from build123d import *

# Parameters (mm, degrees)
F1_DEPTH = 5
F3_DEPTH = 10
F5_DEPTH = 25


with BuildPart() as f1:
    # F0 (on Front) → F1 (new body)
    with BuildSketch(Plane.XZ):
        with BuildLine():
            Line((32.2, -24), (32.2, 24))
            Line((32.2, 24), (6.5, 24))
            Line((6.5, 24), (6.5, 10.8))
            Line((6.5, 10.8), (8.4, 10.8))
            Line((8.4, 10.8), (8.4, 14.8))
            ThreePointArc((8.4, 14.8), (14.9, 21.3), (21.4, 14.8))
            Line((21.4, 14.8), (21.4, 10.8))
            Line((21.4, 10.8), (24.4, 10.8))
            Line((24.4, 10.8), (24.4, -10.8))
            Line((24.4, -10.8), (21.4, -10.8))
            Line((21.4, -10.8), (21.4, -14.8))
            ThreePointArc((21.4, -14.8), (14.9, -21.3), (8.4, -14.8))
            Line((8.4, -14.8), (8.4, -10.8))
            Line((8.4, -10.8), (-8.4, -10.8))
            Line((-8.4, -10.8), (-8.4, -14.8))
            ThreePointArc((-8.4, -14.8), (-14.9, -21.3), (-21.4, -14.8))
            Line((-21.4, -14.8), (-21.4, -10.8))
            Line((-21.4, -10.8), (-24.4, -10.8))
            Line((-24.4, -10.8), (-24.4, 10.8))
            Line((-24.4, 10.8), (-21.4, 10.8))
            Line((-21.4, 10.8), (-21.4, 14.8))
            ThreePointArc((-21.4, 14.8), (-14.9, 21.3), (-8.4, 14.8))
            Line((-8.4, 14.8), (-8.4, 10.8))
            Line((-8.4, 10.8), (-6.5, 10.8))
            Line((-6.5, 10.8), (-6.5, 24))
            Line((-6.5, 24), (-32.2, 24))
            Line((-32.2, 24), (-32.2, -24))
            Line((-32.2, -24), (32.2, -24))
        make_face()
    extrude(amount=F1_DEPTH)

    # F2 (on face) → F3 (join)
    with BuildSketch(Plane(origin=(0, 0, 0), x_dir=(-1, 0, 0), z_dir=(0, 1, 0))):
        with BuildLine():
            Line((24.4, 10.8), (24.4, -10.8))
            Line((24.4, -10.8), (21.4, -10.8))
            Line((21.4, -10.8), (21.4, -14.8))
            ThreePointArc((21.4, -14.8), (14.9, -21.3), (8.4, -14.8))
            Line((8.4, -14.8), (8.4, -10.8))
            Line((8.4, -10.8), (-8.4, -10.8))
            Line((-8.4, -10.8), (-8.4, -14.8))
            ThreePointArc((-8.4, -14.8), (-14.9, -21.3), (-21.4, -14.8))
            Line((-21.4, -14.8), (-21.4, -10.8))
            Line((-21.4, -10.8), (-24.4, -10.8))
            Line((-24.4, -10.8), (-24.4, 10.8))
            Line((-24.4, 10.8), (-21.4, 10.8))
            Line((-21.4, 10.8), (-21.4, 14.8))
            ThreePointArc((-21.4, 14.8), (-14.9, 21.3), (-8.4, 14.8))
            Line((-8.4, 14.8), (-8.4, 10.8))
            Line((-8.4, 10.8), (-6.5, 10.8))
            Line((-6.5, 10.8), (-6.5, 24))
            Line((-6.5, 24), (-32.2, 24))
            Line((-32.2, 24), (-32.2, -24))
            Line((-32.2, -24), (32.2, -24))
            Line((32.2, -24), (32.2, 24))
            Line((32.2, 24), (6.5, 24))
            Line((6.5, 24), (6.5, 10.8))
            Line((6.5, 10.8), (8.4, 10.8))
            Line((8.4, 10.8), (8.4, 14.8))
            ThreePointArc((8.4, 14.8), (14.9, 21.3), (21.4, 14.8))
            Line((21.4, 14.8), (21.4, 10.8))
            Line((21.4, 10.8), (24.4, 10.8))
        make_face()
        with BuildLine():
            Line((21.4, -14.8), (21.4, -10.8))
            Line((21.4, -10.8), (8.4, -10.8))
            Line((8.4, -10.8), (8.4, -14.8))
            ThreePointArc((8.4, -14.8), (14.9, -21.3), (21.4, -14.8))
        make_face()
        with BuildLine():
            Line((-8.4, -14.8), (-8.4, -10.8))
            Line((-8.4, -10.8), (-21.4, -10.8))
            Line((-21.4, -10.8), (-21.4, -14.8))
            ThreePointArc((-21.4, -14.8), (-14.9, -21.3), (-8.4, -14.8))
        make_face()
        with BuildLine():
            Line((8.4, 10.8), (21.4, 10.8))
            Line((21.4, 10.8), (21.4, 14.8))
            ThreePointArc((21.4, 14.8), (14.9, 21.3), (8.4, 14.8))
            Line((8.4, 14.8), (8.4, 10.8))
        make_face()
        with BuildLine():
            Line((-21.4, 10.8), (-8.4, 10.8))
            Line((-8.4, 10.8), (-8.4, 14.8))
            ThreePointArc((-8.4, 14.8), (-14.9, 21.3), (-21.4, 14.8))
            Line((-21.4, 14.8), (-21.4, 10.8))
        make_face()
    extrude(amount=F3_DEPTH)

    # F4 (on face) → F5 (join)
    with BuildSketch(Plane(origin=(0, 10, 0), x_dir=(-1, 0, 0), z_dir=(0, 1, 0))):
        Polygon((32.2, -24), (32.2, 24), (6.5, 24), (6.5, 10.8), (24.4, 10.8), (24.4, -10.8), (-24.4, -10.8), (-24.4, 10.8), (-6.5, 10.8), (-6.5, 24), (-32.2, 24), (-32.2, -24), align=None)
        Polygon((6.5, 10.8), (6.5, 24), (-6.5, 24), (-6.5, 10.8), (-24.4, 10.8), (-24.4, -10.8), (24.4, -10.8), (24.4, 10.8), align=None)
        with BuildLine():
            ThreePointArc((5.5288725662, 5.5), (16.8680666762, 9.6842239514), (24.1, 0))
            ThreePointArc((24.1, 0), (16.8680666762, -9.6842239514), (5.5288725662, -5.5))
            Line((5.5288725662, -5.5), (0, -5.5))
            Line((0, -5.5), (-5.5288725662, -5.5))
            ThreePointArc((-5.5288725662, -5.5), (-24.1, 0), (-5.5288725662, 5.5))
            Line((-5.5288725662, 5.5), (0, 5.5))
            Line((0, 5.5), (5.5288725662, 5.5))
        make_face(mode=Mode.SUBTRACT)
    extrude(amount=F5_DEPTH)


solid = f1.part
Work out the finished part from the listing and answer in its coordinate system (mm). A direction names the side the tool comes from. Give positions to 0.01 mm unless a question says otherwise; leave off trailing zeros. Loops run counter-clockwise (first coordinate to the right, second up) from the corner with the lowest first, then second, coordinate; pieces in that order, holes last. Notation, with made-up numbers: (-34, 18.25) - (15, 18.25) arc R18 cw to (15, 50.25) - close; hole circle Ø2 at (35, 49.5). An arc over 180 degrees is marked (long way). Answer in a Markdown table with one row per item. Add a question column.
Q1. The part is cut by section C-C (x = 19.5). Determine the outline of the cut face in (y, z).
Q2. The part is cut by section D-D (y = 7). Determine the outline of the cut face in (x, z).
Q3. A tool of negligible diameter and unlimited length cuts with its end or side. For faces 3 (the flat face through (0, 22, -5.5)), 4 (the flat face through (-15, 0, 15)), 5 (the flat face through (-32.2, 15, 0)), from which of +Z, -Z, +X, -X, +Y, -Y can it reach the whole face along a straight path? Write none if from no direction.
Q4. Consider line 1 along X through (y, z) = (2, 9.5); line 2 along X through (y, z) = (23.5, 0); line 3 along Z through (x, y) = (14, 15). Determine where each line is inside the solid, lowest interval first.
Q5. This flat-tipped pin is pushed along its axis until it touches: P1, Ø5, axis at x = 12, z = -15, coming from the -Y side. Where does it stop, or does it pass through?
Q6. Determine the mould class of faces 1 (the flat face through (21.4, -2, -13)), 2 (the flat face through (-8, -5, 11)) for opening direction Z: released by +Z, released by -Z, zero draft, split by the parting line, or undercut.
Q7. The part is cut by section A-A (y = 26). Determine the outline of the cut face in (x, z).
Q8. The part is cut by section B-B (z = 8.5). Determine the outline of the cut face in (x, y).
Solution:
| question | item | result |
|---|---|---|
| 1 | outline | (-5, -24) - (35, -24) - (35, -8.47) - (10, -8.47) - (10, -10.8) - (0, -10.8) - (0, -19.39) - (-5, -19.39) - close; (-5, 19.39) - (0, 19.39) - (0, 10.8) - (10, 10.8) - (10, 8.47) - (35, 8.47) - (35, 24) - (-5, 24) - close |
| 2 | outline | (-32.2, -24) - (32.2, -24) - (32.2, 24) - (6.5, 24) - (6.5, 10.8) - (24.4, 10.8) - (24.4, -10.8) - (-24.4, -10.8) - (-24.4, 10.8) - (-6.5, 10.8) - (-6.5, 24) - (-32.2, 24) - close |
| 3 | face 3 | +Y, -Y |
| 3 | face 4 | -Y |
| 3 | face 5 | +Z, -Z, -X, +Y, -Y |
| 4 | line 1 | x = -32.2 to -24.4, 24.4 to 32.2 |
| 4 | line 2 | x = -32.2 to -24.1, 24.1 to 32.2 |
| 4 | line 3 | z = -24 to -10.1, 10.1 to 24 |
| 5 | P1 | stops at y = 0 |
| 6 | face 1 | undercut |
| 6 | face 2 | zero draft |
| 7 | outline | (-32.2, -24) - (32.2, -24) - (32.2, 24) - (-32.2, 24) - close; hole (-5.53, -5.5) - (5.53, -5.5) arc R10.1 ccw (long way) to (5.53, 5.5) - (-5.53, 5.5) arc R10.1 ccw (long way) to start |
| 8 | outline | (-32.2, -5) - (-24.4, -5) - (-24.4, 10) - (-19.46, 10) - (-19.46, 35) - (-32.2, 35) - close; (-8.54, 10) - (8.54, 10) - (8.54, 35) - (-8.54, 35) - close; (19.46, 10) - (24.4, 10) - (24.4, -5) - (32.2, -5) - (32.2, 35) - (19.46, 35) - close |
